Source: CAD feature listing. Evaluate the final solid. Frame: model axes, mm. Face numbers are marked on the shaded views. A direction names the side the tool comes from. Coordinates: 2 decimals unless noted, no trailing zeros. Order: outer loops, then holes, each group sorted by start corner. A loop starts at its lowest first (then second) coordinate and runs counter-clockwise, first axis right, second up. Notation, with made-up numbers: (-32, 62.25) -> (-2, 62.25) arc R26 cw to (-2, 88.25) -> close; hole circle Ø5 at (72, 74.25). An arc over 180 degrees is marked (long way). Write item = value, one per line. Start each with the question number.
Item 1: Section query C-C (y = -1.5). Output: boundary loops of the cut face in (x, z).
Item 2: Section query B-B (x = 4). Output: boundary loops of the cut face in (y, z), then the cut area to 3 significant figures.
Item 3: Mould query, pull axis Y, two halves, no side actions, for the marked faces 4, 5 and 6. Classes: released by +Y, released by -Y, zero draft, split by the parting line, or undercut.
Item 4: Set-up query: the marked faces 1, 2 and 3. Return all of +Z, -Z, +X, -X, +Y, -Y with unobstructed straight access to the full face (end or side cutting, diameter ignored); none if empty.
Item 5: Ray query, line 1 along Y through (x, z) = (0, 1.1); line 2 along X through (y, z) = (3.5, 1.25); line 3 along Y through (x, z) = (-5, 3.25). Return the intervals inside material, ascending. Write a range as [from, to].
Item 6: Section query D-D (y = 2). Output: boundary loops of the cut face in (x, z), then the cut area to 3 significant figures.
Item 7: Contact query for flat-ended pins moving along their axis: pin 1 (1 mm diameter, centred on x = 5, y = -3, fed in from -Z); pin 2 (1 mm diameter, centred on y = -10.5, z = 3.5, fed in from +X); pin 3 (1 mm diameter, centred on x = 4, y = -17.5, fed in from +Z); pin 4 (8.5 mm diameter, centred on x = 1, y = -1, fed in from +Z). Output: stop coordinate, or through.
Item 8: Section query A-A (x = -5.25). Output: boundary loops of the cut face in (y, z), then the cut area to 3 significant figures.
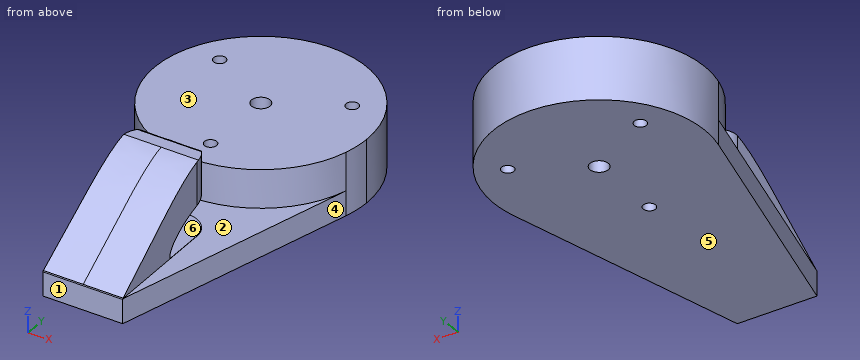
```python
from build123d import *

# Parameters (mm, degrees)
F0_R     = 0.5
F0_R_2   = 0.75
F1_DEPTH = 5.1
F2_DEPTH = 2
F4_DEPTH = 6
F6_DEPTH = 12.5


with BuildPart() as f1:
    # F0 (on Top) → F1 (new body)
    with BuildSketch(Plane.XY):
        with BuildLine():
            ThreePointArc((8.3343568954, -2.1209656149), (8.5333308063, -1.0687681459), (8.6, 0))
            ThreePointArc((8.6, 0), (-1.0687681459, 8.5333308063), (-8.3343568954, -2.1209656149))
            ThreePointArc((-8.3343568954, -2.1209656149), (0, -8.6), (8.3343568954, -2.1209656149))
        make_face()
        with Locations((-5.405664058, 3.1209615991)):
            Circle(F0_R, mode=Mode.SUBTRACT)
        with Locations((0, -6.2419231981)):
            Circle(F0_R, mode=Mode.SUBTRACT)
        Circle(F0_R_2, mode=Mode.SUBTRACT)
        with Locations((5.405664058, 3.1209615991)):
            Circle(F0_R, mode=Mode.SUBTRACT)
    extrude(amount=F1_DEPTH)

    # F0 (on Top) → F2 (join)
    with BuildSketch(Plane.XY):
        with BuildLine():
            ThreePointArc((8.3343568954, -2.1209656149), (0, -8.6), (-8.3343568954, -2.1209656149))
            Line((-8.3343568954, -2.1209656149), (-3.25, -22.1))
            Line((-3.25, -22.1), (3.25, -22.1))
            Line((3.25, -22.1), (8.3343568954, -2.1209656149))
        make_face()
    extrude(amount=F2_DEPTH)

    # F3 (on face) → F4 (join)
    with BuildSketch(Plane.XY.offset(2)):
        with BuildLine():
            Line((-3.0482308868, -12.5577199533), (-3.25, -22.1))
            Line((-3.25, -22.1), (3.25, -22.1))
            Line((3.25, -22.1), (3.0482308868, -12.5577199533))
            ThreePointArc((3.0482308868, -12.5577199533), (2.447863298, -11.1709163612), (1.0486778373, -10.6))
            Line((1.0486778373, -10.6), (-1.0486778373, -10.6))
            ThreePointArc((-1.0486778373, -10.6), (-2.447863298, -11.1709163612), (-3.0482308868, -12.5577199533))
        make_face()
    extrude(amount=F4_DEPTH)

    # F5 (on Right) → F6 (intersect, symmetric)
    with BuildSketch(Plane.YZ):
        with BuildLine():
            add(Edge.make_bspline(
                [(-22.0577802784, 2.0259046448), (-17.8050547421, 4.9004560213), (-14.5293847897, 7.5751652736), (-10.4708936119, 8.5418524459), (-10.5693109534, 4.5828096798), (-13.2662088909, 4.6015626195), (-16.1733651308, 2.8726245308), (-16.0577802784, 2.0259046448)],
                knots=[0, 0, 0, 0, 0.3238992112, 0.4862577355, 0.646782374, 0.8105162215, 1, 1, 1, 1], degree=3))
            Line((-22.0577802784, 2.0259046448), (-23.0374708772, 0))
            Line((-23.0374708772, 0), (-19.6792803642, -1.6239597866))
            Line((-19.6792803642, -1.6239597866), (11.3044586033, -3.4222211689))
            Line((11.3044586033, -3.4222211689), (11.6330533383, 2.2394104473))
            Line((11.6330533383, 2.2394104473), (9.3493293971, 8.4649659693))
            Line((9.3493293971, 8.4649659693), (-3.0461885035, 7.9566333443))
            Line((-3.0461885035, 7.9566333443), (-9.4479173422, 6.1554415151))
            Line((-9.4479173422, 6.1554415151), (-9.5424316823, 4.2449091561))
            Line((-9.5424316823, 4.2449091561), (-10.334789753, 2.0259046448))
            Line((-10.334789753, 2.0259046448), (-16.0577802784, 2.0259046448))
        make_face()
    extrude(amount=F6_DEPTH, both=True, mode=Mode.INTERSECT)


solid = f1.part
```
Computed:
q1.outline = (-8.47, 0) -> (8.47, 0) -> (8.47, 5.1) -> (-8.47, 5.1) -> close
q2.outline = (-19.15, 0) -> (7.61, 0) -> (7.61, 5.1) -> (-7.61, 5.1) -> (-7.61, 2) -> (-19.15, 2) -> close
q2.area = 101 mm^2
q3.face_4 = released by -Y
q3.face_5 = zero draft
q3.face_6 = undercut
q4.face_1 = +Z, -Z, +X, -X, -Y
q4.face_2 = +Z
q4.face_3 = +Z, +X, -X, +Y
q5.line_1 = [-22.1, -6.74], [-5.74, -0.75], [0.75, 8.6]
q5.line_2 = [-7.86, -5.73], [-5.08, 5.08], [5.73, 7.86]
q5.line_3 = [-7, 2.83], [3.41, 7]
q6.outline = (-8.36, 0) -> (8.36, 0) -> (8.36, 5.1) -> (-8.36, 5.1) -> close
q6.area = 85.3 mm^2
q7.pin_1 = 0
q7.pin_2 = through
q7.pin_3 = 2
q7.pin_4 = 5.1
q8.outline = (-14.24, 0) -> (2.65, 0) -> (2.65, 5.1) -> (-6.81, 5.1) -> (-6.81, 2) -> (-14.24, 2) -> close; (3.6, 0) -> (6.81, 0) -> (6.81, 5.1) -> (3.6, 5.1) -> close
q8.area = 79.5 mm^2
